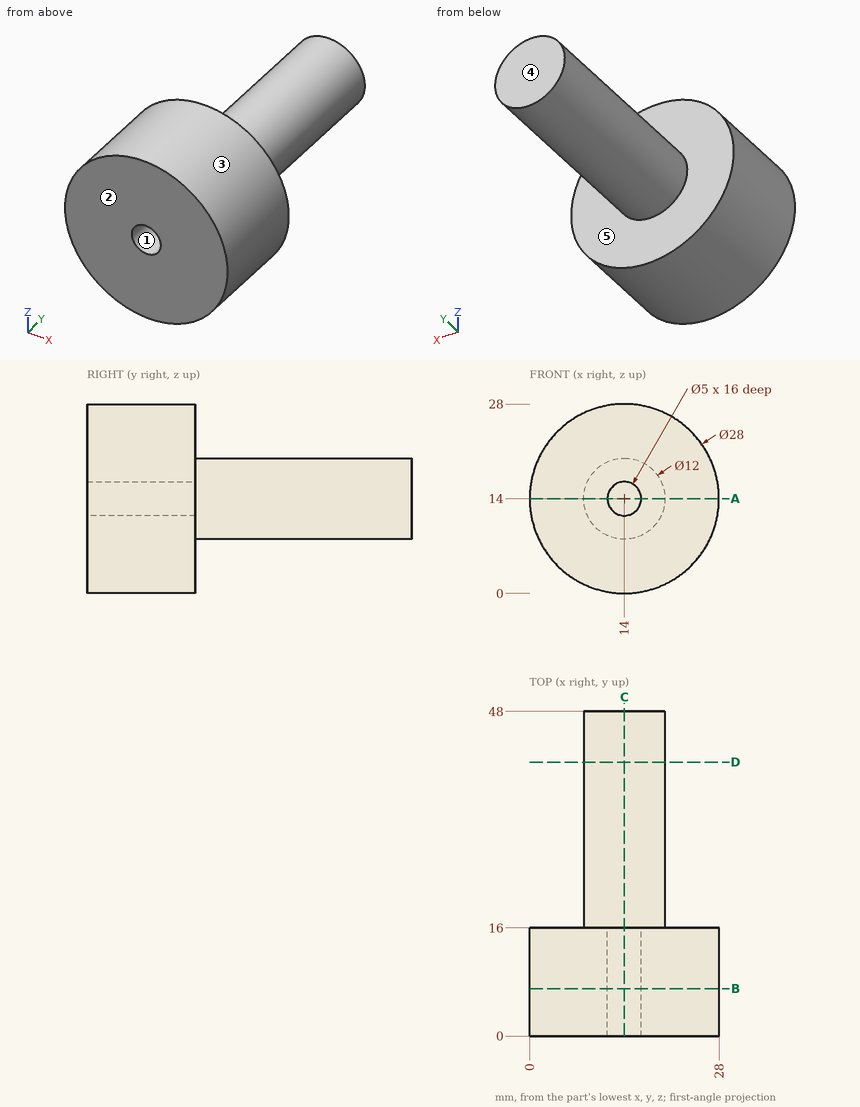
Check sheet for the drawn part. Datum: minimum x, y, z corner. Units: mm. A direction names the side the tool comes from. Round coordinates to 2 decimals unless told otherwise and drop trailing zeros. Loops run counter-clockwise (first coordinate to the right, second up) from the corner with the lowest first, then second, coordinate; pieces in that order, holes last. Notation, with made-up numbers: (0, 4) -> (14, 4) arc R15 cw to (14, 18) -> close; hole circle Ø6 at (18, -23.5). An arc over 180 degrees is marked (long way). Put each result on its own line as item: value. Start each with the question number.
1. Scan lines: probe 1 along X at (y, z) = (9.25, 14); probe 2 along Y at (x, z) = (20.5, 10.25); probe 3 along Z at (x, y) = (22.75, 9.5). Record each from-to range of solid material in increasing order.
2. Section check A-A (z = 14). Enter the section's corners in (x, y), plus the area to 3 significant figures.
3. Section check C-C (x = 14). Enter the section's corners in (y, z).
4. Draft check along Z on the marked faces 1, 2 and 3. Enter one of: +Z half, -Z half, draft (parallel to the pull), parting line (faces both ways), or undercut.
5. Gauge pin test, flat ends, axial feed: pin 1 (6 mm diameter, centred on y = 5.5, z = 9, fed in from -X); pin 2 (10 mm diameter, centred on x = 5, y = 8.5, fed in from -Z); pin 3 (2 mm diameter, centred on x = 9.5, y = 5.5, fed in from -Z). Record the tip position at first contact, or that the pin passes through.
6. Section check B-B (y = 7). Enter the section's corners in (x, z), plus the area to 3 significant figures.
7. Access from +Z, -Z, +X, -X, +Y, -Y to the whole of each face (thin tool, end or side, straight path). Record for the marked faces 4 and 5.
8. Section check D-D (y = 40.5). Enter the section's corners in (x, z), plus the area to 3 significant figures.
Findings:
1. probe 1: x = 0 to 11.5, 16.5 to 28
1. probe 2: y = 0 to 16
1. probe 3: z = 3.07 to 24.93
2. outline: (0, 0) -> (11.5, 0) -> (11.5, 16) -> (16.5, 16) -> (16.5, 0) -> (28, 0) -> (28, 16) -> (20, 16) -> (20, 48) -> (8, 48) -> (8, 16) -> (0, 16) -> close
2. area: 752 mm^2
3. outline: (0, 0) -> (16, 0) -> (16, 8) -> (48, 8) -> (48, 20) -> (16, 20) -> (16, 28) -> (0, 28) -> (0, 16.5) -> (16, 16.5) -> (16, 11.5) -> (0, 11.5) -> close
4. face 1: undercut
4. face 2: draft
4. face 3: parting line
5. pin 1: stops at x = 0.14
5. pin 2: stops at z = 0.58
5. pin 3: stops at z = 0.44
6. outline: circle Ø28 at (14, 14); hole circle Ø5 at (14, 14)
6. area: 596 mm^2
7. face 4: +Z, -Z, +X, -X, +Y
7. face 5: +Y
8. outline: circle Ø12 at (14, 14)
8. area: 113 mm^2
